Answer from the drawing. Dimensions are ordinates in mm from the lowest x, y and z of the part. Give positions to 0.01 mm unless a question says otherwise; leave off trailing zeros. Loops run counter-clockwise (first coordinate to the right, second up) from the corner with the lowest first, then second, coordinate; pieces in that order, holes last. Notation, with made-up numbers: (56, -36.5) - (108, -36.5) arc R26 ccw to (108, -21.5) - close; hole circle Ø8 at (75, 47). An arc over 180 degrees is marked (long way). Put each result on its own line as item: value. Start each with the question number.
1. A cutting plane is placed at A-A, the plane z = 111. Determine the outline of the cut face in (x, y), plus the area to 3 significant figures.
2. Given pin 1 Ø12 at (x, z) = (3.5, 95.5) entering from +Y; pin 2 Ø11 at (x, y) = (11.5, 13.5) entering from -Z; pin 3 Ø9 at (x, y) = (12.5, 12.5) entering from +Z; pin 4 Ø1.5 at (x, z) = (6, 78.5) entering from -Y, each flat-ended and moving along its own axis, determine where each tip first touches the part or whether it passes through.
3. A cutting plane is placed at D-D, the plane z = 46. Determine the outline of the cut face in (x, y).
4. Consider L1, parallel to Y at x = 12.5, z = 11.5; L2, parallel to X at y = 16.25, z = 96.5; L3, parallel to Y at x = 10.25, z = 19. Determine where each line is inside the solid, lowest interval first. Write a range as from..to.
5. A cutting plane is placed at B-B, the plane x = 12.5. Determine the outline of the cut face in (y, z).
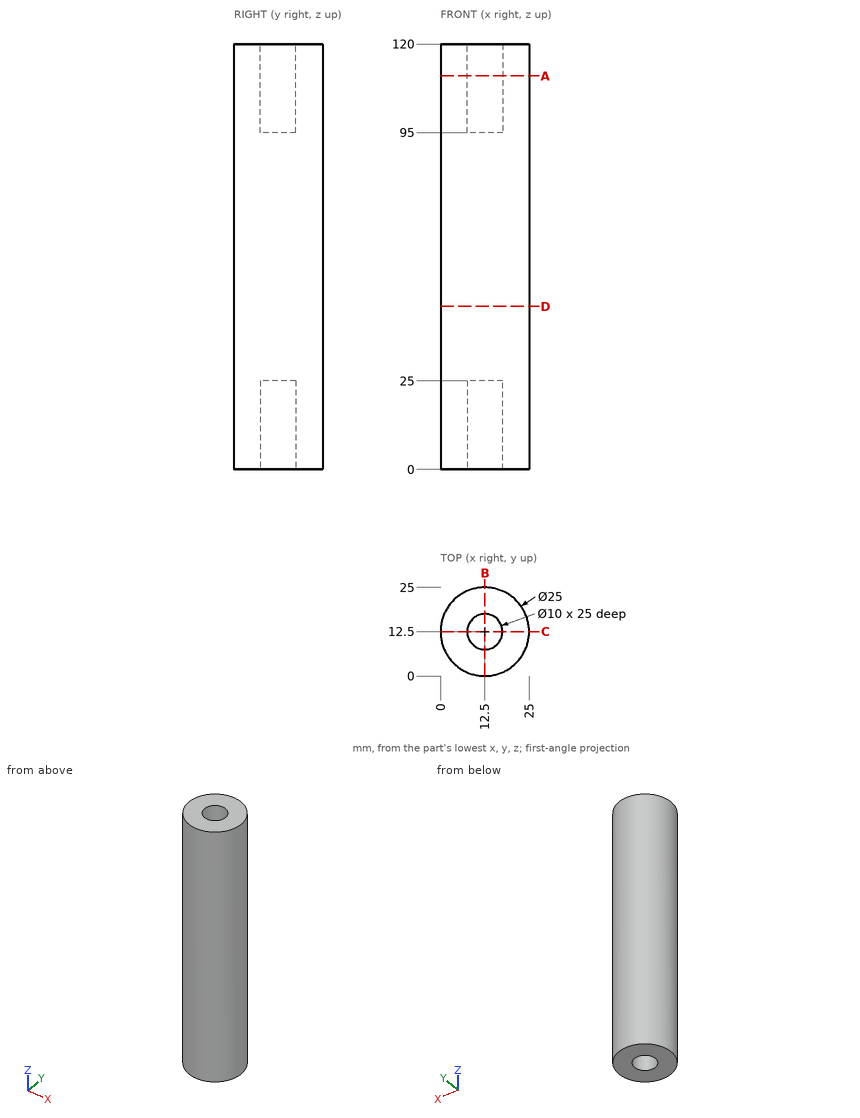
Return value:
1. outline: circle Ø25 at (12.5, 12.5); hole circle Ø10 at (12.5, 12.5)
1. area: 412 mm2
2. pin 1: stops at y = 24.63
2. pin 2: stops at z = 0
2. pin 3: stops at z = 95
2. pin 4: stops at y = 1.4
3. outline: circle Ø25 at (12.5, 12.5)
4. L1: y = 0..7.5, 17.5..25
4. L2: x = 0.58..9.19, 15.81..24.42
4. L3: y = 0.2..8.03, 16.97..24.8
5. outline: (0, 0) - (7.5, 0) - (7.5, 25) - (17.5, 25) - (17.5, 0) - (25, 0) - (25, 120) - (17.5, 120) - (17.5, 95) - (7.5, 95) - (7.5, 120) - (0, 120) - close
